Answer from the drawing. Dimensions are ordinates in mm from the lowest x, y and z of the part. A direction names the side the tool comes from. Coordinates: 2 decimals unless noted, no trailing zeros. Order: outer loops, then holes, each group sorted by start corner. A loop starts at its lowest first (then second) coordinate and runs counter-clockwise, first axis right, second up.
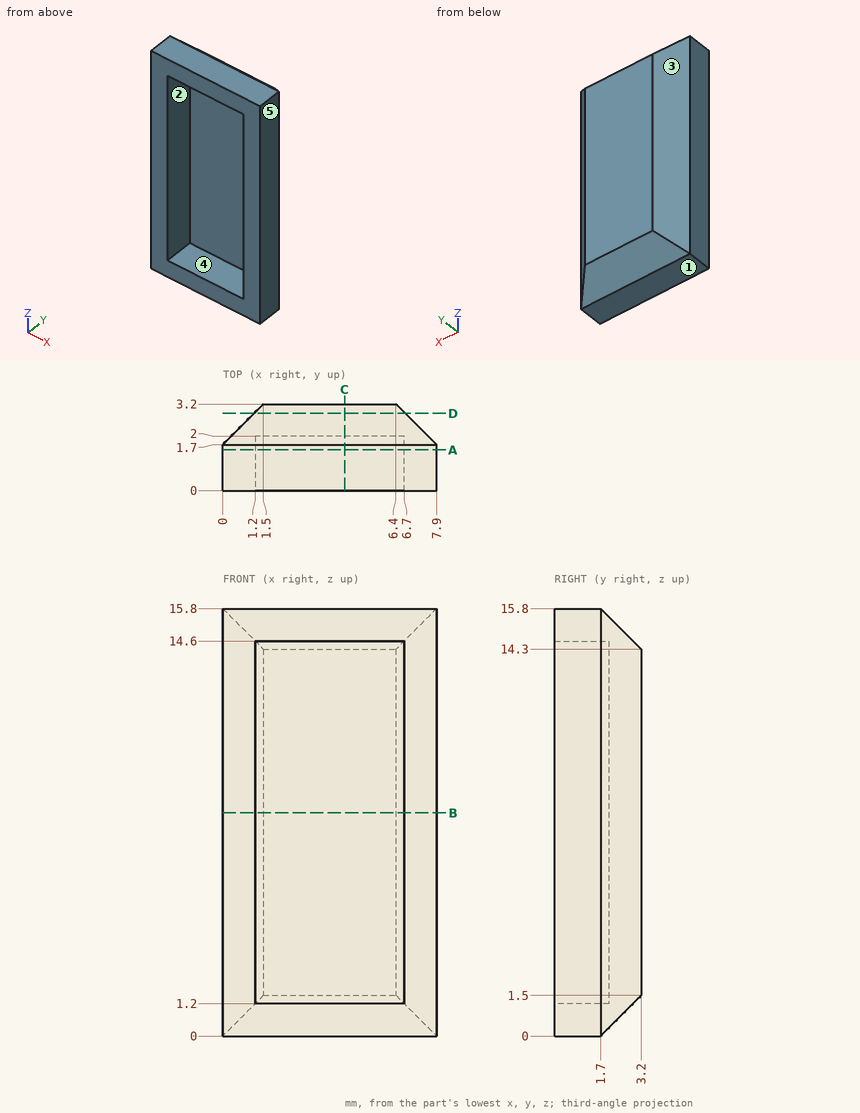
1. The part is cut by section C-C (x = 4.5). Determine the outline of the cut face in (y, z), plus the area to 3 significant figures.
2. The mould has two halves that part along Z. Classify the marked faces 1, 2 and 3: released by +Z, released by -Z, zero draft, split by the parting line, or undercut.
3. The part is cut by section D-D (y = 2.85). Determine the outline of the cut face in (x, z).
4. For the marked faces 4 and 5, determine the directions among +Z, -Z, +X, -X, +Y, -Y from which every point of the face is accessible in a straight line to the end or side of a thin tool.
5. The part is cut by section A-A (y = 1.5). Determine the outline of the cut face in (x, z).
6. Consider probe 1 along X at (y, z) = (1.15, 14); probe 2 along Z at (x, y) = (4.25, 1.05); probe 3 along Y at (x, z) = (4.25, 12.25). Determine where each line is inside the solid, lowest interval first.
7. The part is cut by section B-B (z = 8.25). Determine the outline of the cut face in (x, y), plus the area to 3 significant figures.
Worked out:
1. outline: (0, 0) - (1.7, 0) - (3.2, 1.5) - (3.2, 14.3) - (1.7, 15.8) - (0, 15.8) - (0, 14.6) - (2, 14.6) - (2, 1.2) - (0, 1.2) - close
1. area: 21.5 mm2
2. face 1: released by -Z
2. face 2: undercut
2. face 3: zero draft
3. outline: (1.15, 1.15) - (6.75, 1.15) - (6.75, 14.65) - (1.15, 14.65) - close
4. face 4: -Y
4. face 5: +Z, -Z, +X, +Y, -Y
5. outline: (0, 0) - (7.9, 0) - (7.9, 15.8) - (0, 15.8) - close; hole (1.2, 1.2) - (6.7, 1.2) - (6.7, 14.6) - (1.2, 14.6) - close
6. probe 1: x = 0 to 1.2, 6.7 to 7.9
6. probe 2: z = 0 to 1.2, 14.6 to 15.8
6. probe 3: y = 2 to 3.2
7. outline: (0, 0) - (1.2, 0) - (1.2, 2) - (6.7, 2) - (6.7, 0) - (7.9, 0) - (7.9, 1.7) - (6.4, 3.2) - (1.5, 3.2) - (0, 1.7) - close
7. area: 12.0 mm2
